Input: part model. Units: mm. Frame: model coordinates. A direction names the side the tool comes from. Round coordinates to 2 decimals unless told otherwise and drop trailing zeros. Write each loop counter-clockwise with the first axis right and the second up, starting at its lowest first coordinate (ties: lowest second). Pieces come first, ordered by that corner, then holes. Notation, with made-up numbers: (50.5, -34.5) - (60.5, -34.5) arc R15 cw to (60.5, -21.5) - close; hole circle Ø8 at (56, 41). An arc over 180 degrees is marked (long way). One line per item, written item: value. Start each with the question number.
```python
from build123d import *

# Parameters (mm, degrees)
BOSS_EXTRUDE1_DEPTH      = 70
BOSS_EXTRUDE1_DEPTH_BACK = 30
CUT_EXTRUDE1_REACH       = 92
SKETCH3_R                = 1.7
SKETCH3_R_2              = 17.5
SKETCH3_R_3              = 5.1
SKETCH3_R_4              = 3.8
CUT_EXTRUDE2_REACH       = 92
SKETCH4_R                = 5
SKETCH4_R_2              = 3.4
SKETCH5_W                = 20
SKETCH5_H                = 20
CUT_EXTRUDE3_DEPTH       = 1
CUT_EXTRUDE3_DEPTH_BACK  = 91
SKETCH6_W                = 20
SKETCH6_H                = 20
CUT_EXTRUDE4_DEPTH       = 91
SKETCH7_W                = 3
SKETCH7_H                = 20
SKETCH7_W_2              = 20
SKETCH7_H_2              = 3
CUT_EXTRUDE5_DEPTH       = 81
BOSS_EXTRUDE2_DEPTH      = 80


with BuildPart() as part:
    # Sketch2 → Boss-Extrude1 (new body, two sides)
    with BuildSketch(Plane(origin=(0, 0, 0), x_dir=(0, 0, -1), z_dir=(1, 0, 0))) as boss_extrude1_sk:
        with BuildLine():
            Line((3434.65392981, 139.447907294), (3384.65392981, 139.447907294))
            ThreePointArc((3384.65392981, 139.447907294), (3370.511794186, 133.590042917), (3364.65392981, 119.447907294))
            Line((3364.65392981, 119.447907294), (3364.65392981, 69.447907294))
            ThreePointArc((3364.65392981, 69.447907294), (3370.511794186, 55.30577167), (3384.65392981, 49.447907294))
            Line((3384.65392981, 49.447907294), (3434.65392981, 49.447907294))
            ThreePointArc((3434.65392981, 49.447907294), (3448.796065434, 55.30577167), (3454.65392981, 69.447907294))
            Line((3454.65392981, 69.447907294), (3454.65392981, 119.447907294))
            ThreePointArc((3454.65392981, 119.447907294), (3448.796065434, 133.590042917), (3434.65392981, 139.447907294))
        make_face()
        with BuildLine():
            Line((3434.65392981, 129.447907294), (3384.65392981, 129.447907294))
            ThreePointArc((3384.65392981, 129.447907294), (3377.582861998, 126.518975106), (3374.65392981, 119.447907294))
            Line((3374.65392981, 119.447907294), (3374.65392981, 69.447907294))
            ThreePointArc((3374.65392981, 69.447907294), (3377.582861998, 62.376839482), (3384.65392981, 59.447907294))
            Line((3384.65392981, 59.447907294), (3434.65392981, 59.447907294))
            ThreePointArc((3434.65392981, 59.447907294), (3441.724997622, 62.376839482), (3444.65392981, 69.447907294))
            Line((3444.65392981, 69.447907294), (3444.65392981, 119.447907294))
            ThreePointArc((3444.65392981, 119.447907294), (3441.724997622, 126.518975106), (3434.65392981, 129.447907294))
        make_face(mode=Mode.SUBTRACT)
    extrude(amount=BOSS_EXTRUDE1_DEPTH)
    extrude(boss_extrude1_sk.sketch, amount=-BOSS_EXTRUDE1_DEPTH_BACK)

    # Sketch3 → Cut-Extrude1 (cut, up to next)
    with BuildSketch(Plane.XY.offset(-3364.65392981), mode=Mode.PRIVATE) as cut_extrude1_sk1:
        with Locations((15.499999999, 78.947907294)):
            Circle(SKETCH3_R)
    cut_extrude1_tool1 = extrude(cut_extrude1_sk1.sketch, amount=-CUT_EXTRUDE1_REACH, mode=Mode.PRIVATE) & part.part
    add(cut_extrude1_tool1.solids().sort_by_distance((15.5, 78.947907, -3364.65393))[0], mode=Mode.SUBTRACT)
    # Sketch3 → Cut-Extrude1 (cut, up to next)
    with BuildSketch(Plane.XY.offset(-3364.65392981), mode=Mode.PRIVATE) as cut_extrude1_sk2:
        with Locations((15.499999999, 109.947907294)):
            Circle(SKETCH3_R)
    cut_extrude1_tool2 = extrude(cut_extrude1_sk2.sketch, amount=-CUT_EXTRUDE1_REACH, mode=Mode.PRIVATE) & part.part
    add(cut_extrude1_tool2.solids().sort_by_distance((15.5, 109.947907, -3364.65393))[0], mode=Mode.SUBTRACT)
    # Sketch3 → Cut-Extrude1 (cut, up to next)
    with BuildSketch(Plane.XY.offset(-3364.65392981), mode=Mode.PRIVATE) as cut_extrude1_sk3:
        with Locations((-15.500000001, 109.947907294)):
            Circle(SKETCH3_R)
    cut_extrude1_tool3 = extrude(cut_extrude1_sk3.sketch, amount=-CUT_EXTRUDE1_REACH, mode=Mode.PRIVATE) & part.part
    add(cut_extrude1_tool3.solids().sort_by_distance((-15.5, 109.947907, -3364.65393))[0], mode=Mode.SUBTRACT)
    # Sketch3 → Cut-Extrude1 (cut, up to next)
    with BuildSketch(Plane.XY.offset(-3364.65392981), mode=Mode.PRIVATE) as cut_extrude1_sk4:
        with Locations((-15.500000001, 78.947907294)):
            Circle(SKETCH3_R)
    cut_extrude1_tool4 = extrude(cut_extrude1_sk4.sketch, amount=-CUT_EXTRUDE1_REACH, mode=Mode.PRIVATE) & part.part
    add(cut_extrude1_tool4.solids().sort_by_distance((-15.5, 78.947907, -3364.65393))[0], mode=Mode.SUBTRACT)
    # Sketch3 → Cut-Extrude1 (cut, up to next)
    with BuildSketch(Plane.XY.offset(-3364.65392981), mode=Mode.PRIVATE) as cut_extrude1_sk5:
        with Locations((0, 94.447907293)):
            Circle(SKETCH3_R_2)
    cut_extrude1_tool5 = extrude(cut_extrude1_sk5.sketch, amount=-CUT_EXTRUDE1_REACH, mode=Mode.PRIVATE) & part.part
    add(cut_extrude1_tool5.solids().sort_by_distance((0, 94.447907, -3364.65393))[0], mode=Mode.SUBTRACT)
    # Sketch3 → Cut-Extrude1 (cut, up to next)
    with BuildSketch(Plane.XY.offset(-3364.65392981), mode=Mode.PRIVATE) as cut_extrude1_sk6:
        with Locations((34.999999999, 94.447907294)):
            Circle(SKETCH3_R_3)
    cut_extrude1_tool6 = extrude(cut_extrude1_sk6.sketch, amount=-CUT_EXTRUDE1_REACH, mode=Mode.PRIVATE) & part.part
    add(cut_extrude1_tool6.solids().sort_by_distance((35, 94.447907, -3364.65393))[0], mode=Mode.SUBTRACT)
    # Sketch3 → Cut-Extrude1 (cut, up to next)
    with BuildSketch(Plane.XY.offset(-3364.65392981), mode=Mode.PRIVATE) as cut_extrude1_sk7:
        with Locations((35, 78.447907293)):
            Circle(SKETCH3_R_4)
    cut_extrude1_tool7 = extrude(cut_extrude1_sk7.sketch, amount=-CUT_EXTRUDE1_REACH, mode=Mode.PRIVATE) & part.part
    add(cut_extrude1_tool7.solids().sort_by_distance((35, 78.447907, -3364.65393))[0], mode=Mode.SUBTRACT)
    # Sketch3 → Cut-Extrude1 (cut, up to next)
    with BuildSketch(Plane.XY.offset(-3364.65392981), mode=Mode.PRIVATE) as cut_extrude1_sk8:
        with Locations((35, 110.447907293)):
            Circle(SKETCH3_R_4)
    cut_extrude1_tool8 = extrude(cut_extrude1_sk8.sketch, amount=-CUT_EXTRUDE1_REACH, mode=Mode.PRIVATE) & part.part
    add(cut_extrude1_tool8.solids().sort_by_distance((35, 110.447907, -3364.65393))[0], mode=Mode.SUBTRACT)

    # Sketch4 → Cut-Extrude2 (cut, up to next)
    with BuildSketch(Plane(origin=(0, 139.447907294, 0), x_dir=(1, 0, 0), z_dir=(0, 1, 0)), mode=Mode.PRIVATE) as cut_extrude2_sk1:
        with Locations((15.6, 3409.65392981)):
            Circle(SKETCH4_R)
    cut_extrude2_tool1 = extrude(cut_extrude2_sk1.sketch, amount=-CUT_EXTRUDE2_REACH, mode=Mode.PRIVATE) & part.part
    add(cut_extrude2_tool1.solids().sort_by_distance((15.6, 139.447907, -3409.65393))[0], mode=Mode.SUBTRACT)
    # Sketch4 → Cut-Extrude2 (cut, up to next)
    with BuildSketch(Plane(origin=(0, 139.447907294, 0), x_dir=(1, 0, 0), z_dir=(0, 1, 0)), mode=Mode.PRIVATE) as cut_extrude2_sk2:
        with Locations((50.6, 3409.65392981)):
            Circle(SKETCH4_R)
    cut_extrude2_tool2 = extrude(cut_extrude2_sk2.sketch, amount=-CUT_EXTRUDE2_REACH, mode=Mode.PRIVATE) & part.part
    add(cut_extrude2_tool2.solids().sort_by_distance((50.6, 139.447907, -3409.65393))[0], mode=Mode.SUBTRACT)
    # Sketch4 → Cut-Extrude2 (cut, up to next)
    with BuildSketch(Plane(origin=(0, 139.447907294, 0), x_dir=(1, 0, 0), z_dir=(0, 1, 0)), mode=Mode.PRIVATE) as cut_extrude2_sk3:
        with Locations((50.6, 3425.65392981)):
            Circle(SKETCH4_R_2)
    cut_extrude2_tool3 = extrude(cut_extrude2_sk3.sketch, amount=-CUT_EXTRUDE2_REACH, mode=Mode.PRIVATE) & part.part
    add(cut_extrude2_tool3.solids().sort_by_distance((50.6, 139.447907, -3425.65393))[0], mode=Mode.SUBTRACT)
    # Sketch4 → Cut-Extrude2 (cut, up to next)
    with BuildSketch(Plane(origin=(0, 139.447907294, 0), x_dir=(1, 0, 0), z_dir=(0, 1, 0)), mode=Mode.PRIVATE) as cut_extrude2_sk4:
        with Locations((50.6, 3393.65392981)):
            Circle(SKETCH4_R_2)
    cut_extrude2_tool4 = extrude(cut_extrude2_sk4.sketch, amount=-CUT_EXTRUDE2_REACH, mode=Mode.PRIVATE) & part.part
    add(cut_extrude2_tool4.solids().sort_by_distance((50.6, 139.447907, -3393.65393))[0], mode=Mode.SUBTRACT)
    # Sketch4 → Cut-Extrude2 (cut, up to next)
    with BuildSketch(Plane(origin=(0, 139.447907294, 0), x_dir=(1, 0, 0), z_dir=(0, 1, 0)), mode=Mode.PRIVATE) as cut_extrude2_sk5:
        with Locations((15.6, 3425.65392981)):
            Circle(SKETCH4_R_2)
    cut_extrude2_tool5 = extrude(cut_extrude2_sk5.sketch, amount=-CUT_EXTRUDE2_REACH, mode=Mode.PRIVATE) & part.part
    add(cut_extrude2_tool5.solids().sort_by_distance((15.6, 139.447907, -3425.65393))[0], mode=Mode.SUBTRACT)
    # Sketch4 → Cut-Extrude2 (cut, up to next)
    with BuildSketch(Plane(origin=(0, 139.447907294, 0), x_dir=(1, 0, 0), z_dir=(0, 1, 0)), mode=Mode.PRIVATE) as cut_extrude2_sk6:
        with Locations((15.6, 3393.65392981)):
            Circle(SKETCH4_R_2)
    cut_extrude2_tool6 = extrude(cut_extrude2_sk6.sketch, amount=-CUT_EXTRUDE2_REACH, mode=Mode.PRIVATE) & part.part
    add(cut_extrude2_tool6.solids().sort_by_distance((15.6, 139.447907, -3393.65393))[0], mode=Mode.SUBTRACT)

    # Sketch5 → Cut-Extrude3 (cut, two sides)
    with BuildSketch(Plane.XY.offset(-3364.65392981)) as cut_extrude3_sk:
        with Locations((-20, 59.447907294)):
            Rectangle(SKETCH5_W, SKETCH5_H)
    extrude(amount=CUT_EXTRUDE3_DEPTH, mode=Mode.SUBTRACT)
    extrude(cut_extrude3_sk.sketch, amount=-CUT_EXTRUDE3_DEPTH_BACK, mode=Mode.SUBTRACT)

    # Sketch6 → Cut-Extrude4 (cut, through all)
    with BuildSketch(Plane(origin=(0, 139.447907294, 0), x_dir=(1, 0, 0), z_dir=(0, 1, 0))):
        with Locations((-20, 3444.65392981)):
            Rectangle(SKETCH6_W, SKETCH6_H)
    extrude(amount=-CUT_EXTRUDE4_DEPTH, mode=Mode.SUBTRACT)

    # Sketch7 → Cut-Extrude5 (cut, through all)
    with BuildSketch(Plane.ZY.offset(10)):
        with BuildLine():
            Line((-3447.65392981, 69.447907294), (-3454.65392981, 69.447907294))
            ThreePointArc((-3454.65392981, 69.447907294), (-3448.796065434, 55.30577167), (-3434.65392981, 49.447907294))
            Line((-3434.65392981, 49.447907294), (-3434.65392981, 56.447907294))
            Line((-3434.65392981, 56.447907294), (-3434.65392981, 59.447907294))
            ThreePointArc((-3434.65392981, 59.447907294), (-3441.724997622, 62.376839482), (-3444.65392981, 69.447907294))
            Line((-3444.65392981, 69.447907294), (-3447.65392981, 69.447907294))
        make_face()
        with Locations((-3446.15392981, 79.447907294)):
            Rectangle(SKETCH7_W, SKETCH7_H)
        with Locations((-3424.65392981, 57.947907294)):
            Rectangle(SKETCH7_W_2, SKETCH7_H_2)
    extrude(amount=-CUT_EXTRUDE5_DEPTH, mode=Mode.SUBTRACT)

    # Sketch8 → Boss-Extrude2 (add)
    with BuildSketch(Plane.ZY.offset(10)):
        with BuildLine():
            Line((-3454.65392981, 79.447907294), (-3434.65392981, 79.447907294))
            ThreePointArc((-3434.65392981, 79.447907294), (-3427.582861998, 76.518975106), (-3424.65392981, 69.447907294))
            Line((-3424.65392981, 69.447907294), (-3424.65392981, 49.447907294))
            Line((-3424.65392981, 49.447907294), (-3434.65392981, 49.447907294))
            Line((-3434.65392981, 49.447907294), (-3434.65392981, 69.447907294))
            Line((-3434.65392981, 69.447907294), (-3454.65392981, 69.447907294))
            Line((-3454.65392981, 69.447907294), (-3454.65392981, 79.447907294))
        make_face()
    extrude(amount=-BOSS_EXTRUDE2_DEPTH)


solid = part.part
```
Q1. Cut plane A-A, the plane y = 68. Output: boundary loops of the cut face in (x, z), and give its area (3 significant figures).
Q2. Cut plane B-B, the plane x = 35. Count the separate pieces of the cut face and the enclosed holes in it, and give its area (3 significant figures).
Q3. Cut plane C-C, the plane z = -3441. Output: boundary loops of the cut face in (x, y), and give its area (3 significant figures).
Q4. Material intervals for probe 1 along Z at (x, y) = (23.5, 79.5); probe 2 along Z at (x, y) = (-4, 114); probe 3 along Y at (x, z) = (53, -3435), sorted ascending. Write a range as from..to.
Q5. Contact query for flat-ended pins moving along their axis: pin 1 Ø6.5 at (x, y) = (25, 66) entering from +Z; pin 2 Ø1.5 at (x, z) = (-19, -3393) entering from -Y; pin 3 Ø4.5 at (x, y) = (-15.5, 78.95) entering from -Z. Output: stop coordinate, or through.
Q6. Access query for faces 4 (the flat face through (-20, 69.448, -3370)), 5 (the flat face through (29, 84, -3447.654)), 6 (the cylindrical face through (50, 135, -3429)). Directions: +Z, -Z, +X, -X, +Y, -Y. A direction counts if a zero-diameter tool reaches every point of the face in a straight line with its end or side. Return the directions, or none.
Q7. Pull-direction query (Z, two-part tool) for faces 1 (the flat face through (21, 95, -3374.654)), 2 (the cylindrical face through (30.56, 55.46, -3370.36)), 3 (the flat face through (-20, 135, -3434.654)); classes: pulls with the +Z half, pulls with the -Z half, needs draft (parallel to the pull), parting line crosses it, or undercut.
A:
1. outline: (-10, -3434.65) - (70, -3434.65) - (70, -3424.65) - (-10, -3424.65) - close; (-10, -3374.76) - (70, -3374.76) - (70, -3364.71) - (-10, -3364.71) - close
1. area: 1,600 mm²
2. separate pieces: 3
2. enclosed holes: 0
2. area: 2,670 mm²
3. outline: (-10, 69.45) - (70, 69.45) - (70, 79.45) - (-10, 79.45) - close; (-10, 127.18) - (70, 127.18) - (70, 138.41) - (-10, 138.41) - close
3. area: 1,700 mm²
4. probe 1: z = -3454.65..-3447.65, -3374.65..-3364.65
4. probe 2: z = -3454.65..-3444.65, -3374.65..-3364.65
4. probe 3: y = 69.45..79.45, 129.44..139.44
5. pin 1: stops at z = -3364.65
5. pin 2: stops at y = 129.45
5. pin 3: stops at z = -3374.65
6. face 4: +Z, -Z, -X, -Y
6. face 5: +X, -X
6. face 6: +Y
7. face 1: undercut
7. face 2: pulls with the +Z half
7. face 3: pulls with the -Z half
